Source: three-view drawing plus pictorial views. Frame: mm from the lowest corner of the part. Coordinates: 2 decimals unless noted, no trailing zeros. Order: outer loops, then holes, each group sorted by start corner. A loop starts at its lowest first (then second) coordinate and runs counter-clockwise, first axis right, second up. Notation, with made-up numbers: (-31, -27) -> (-14, -27) arc R13 cw to (-14, -3) -> close; hole circle Ø4 at (48, -8). An arc over 180 degrees is marked (long way). Use one line per item in the form item = value. Start each with the question number.
1) Ray query, line 1 along X through (y, z) = (10, 16.3); line 2 along X through (y, z) = (9.25, 3.5); line 3 along Z through (x, y) = (23.5, 10). Return the intervals inside material, ascending.
2) Draft query along X for the marked faces 1, 2 and 3. Return one class per face: pulls with the +X half, pulls with the -X half, needs draft (parallel to the pull), parting line crosses it, or undercut.
3) Section query B-B on y = 10. Output: boundary loops of the cut face in (x, z).
4) Section query D-D on y = 6. Output: boundary loops of the cut face in (x, z).
5) Pin query (flat end, axial travel): pin 1 (3.5 mm diameter, centred on x = 6, y = 10, fed in from +Z); pin 2 (4 mm diameter, centred on x = 16, z = 7.5, fed in from -Y); pin 3 (2 mm diameter, centred on x = 5, z = 2, fed in from +Y); pin 4 (4 mm diameter, centred on x = 33, z = 13, fed in from -Y). Return the tip coordinate at first contact, or that it passes through.
6) Section query C-C on x = 33. Output: boundary loops of the cut face in (y, z).
7) Section query A-A on z = 10. Output: boundary loops of the cut face in (x, y), then the cut area to 3 significant figures.
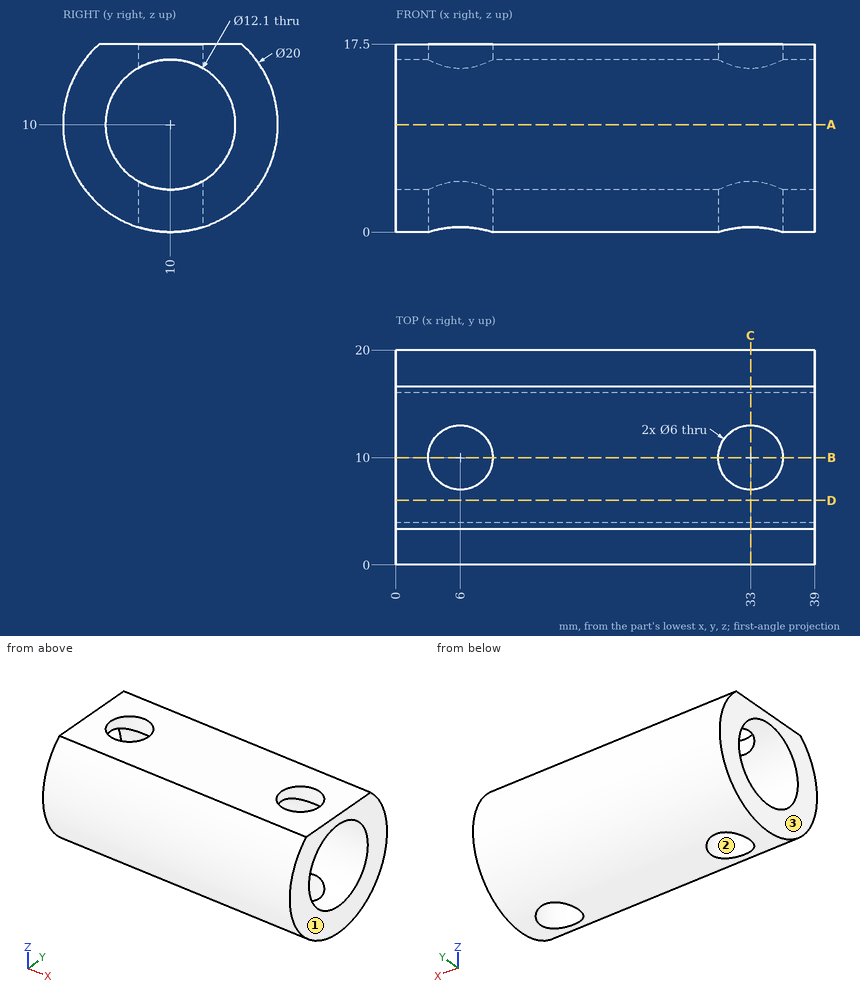
Answers below:
q1.line_1 = 0 to 3, 9 to 30, 36 to 39
q1.line_2 = 0 to 3.1, 8.9 to 30.1, 35.9 to 39
q1.line_3 = 0 to 3.95, 16.05 to 17.5
q2.face_1 = pulls with the +X half
q2.face_2 = undercut
q2.face_3 = pulls with the -X half
q3.outline = (0, 0) -> (3, 0) -> (3, 3.95) -> (0, 3.95) -> close; (0, 16.05) -> (3, 16.05) -> (3, 17.5) -> (0, 17.5) -> close; (9, 0) -> (30, 0) -> (30, 3.95) -> (9, 3.95) -> close; (9, 16.05) -> (30, 16.05) -> (30, 17.5) -> (9, 17.5) -> close; (36, 0) -> (39, 0) -> (39, 3.95) -> (36, 3.95) -> close; (36, 16.05) -> (39, 16.05) -> (39, 17.5) -> (36, 17.5) -> close
q4.outline = (0, 0.83) -> (39, 0.83) -> (39, 5.46) -> (0, 5.46) -> close; (0, 14.54) -> (39, 14.54) -> (39, 17.5) -> (0, 17.5) -> close
q5.pin_1 = through
q5.pin_2 = 0.01
q5.pin_3 = 17.14
q5.pin_4 = 0.05
q6.outline = (3.39, 17.5) arc R10 ccw to (7, 0.46) -> (7, 4.75) arc R6.05 cw to (7, 15.25) -> (7, 17.5) -> close; (13, 0.46) arc R10 ccw to (16.61, 17.5) -> (13, 17.5) -> (13, 15.25) arc R6.05 cw to (13, 4.75) -> close
q7.outline = (0, 0) -> (39, 0) -> (39, 3.95) -> (0, 3.95) -> close; (0, 16.05) -> (39, 16.05) -> (39, 20) -> (0, 20) -> close
q7.area = 308 mm^2
